from build123d import *

# Parameters (mm, degrees)
F1_DEPTH  = 55
F3_DEPTH  = 30
F4_R      = 3
F5_DEPTH  = 25
F6_R      = 12.5
F7_DEPTH  = 25
F8_R      = 15.1
F9_DEPTH  = 38
F10_R     = 15.1
F11_DEPTH = 8
F12_R     = 6.5
F13_DEPTH = 17
F14_R     = 10


with BuildPart() as f1:
    # F0 (on Front) → F1 (new body)
    with BuildSketch(Plane.XZ):
        with BuildLine():
            Line((-23.699999, 23.799999), (-23.699999, 23.558845))
            Line((-23.699999, 23.558845), (-24.369059, 22.399999))
            Line((-24.369059, 22.399999), (-23.699999, 21.241153))
            Line((-23.699999, 21.241153), (-23.699999, -21.000001))
            ThreePointArc((-23.699999, -21.000001), (-22.001218, -25.10122), (-17.899999, -26.8))
            Line((-17.899999, -26.8), (15.100001, -26.8))
            ThreePointArc((15.100001, -26.8), (19.20122, -25.10122), (20.9, -21.000001))
            Line((20.9, -21.000001), (20.9, -4.000001))
            ThreePointArc((20.9, -4.000001), (21.251472, -3.151472), (22.100001, -2.8))
            Line((22.100001, -2.8), (22.9, -2.8))
            Line((22.9, -2.8), (22.9, 2.799999))
            Line((22.9, 2.799999), (22.100001, 2.799999))
            ThreePointArc((22.100001, 2.799999), (21.251472, 3.151471), (20.9, 3.999999))
            Line((20.9, 3.999999), (20.9, 11.499999))
            ThreePointArc((20.9, 11.499999), (21.397919, 12.702081), (22.600001, 13.2))
            Line((22.600001, 13.2), (23.100001, 13.2))
            ThreePointArc((23.100001, 13.2), (23.665686, 13.434314), (23.9, 13.999999))
            Line((23.9, 13.999999), (23.9, 21.241153))
            Line((23.9, 21.241153), (24.56906, 22.399999))
            Line((24.56906, 22.399999), (23.9, 23.558845))
            Line((23.9, 23.558845), (23.9, 23.799999))
            Line((23.9, 23.799999), (-23.699999, 23.799999))
        make_face()
    extrude(amount=F1_DEPTH)

    # F2 (on face) → F3 (cut)
    with BuildSketch(Plane.XZ.offset(55)):
        with BuildLine():
            Line((15.9, 11.457851), (26.682628, 11.457851))
            Line((26.682628, 11.457851), (26.682628, 26.709846))
            Line((26.682628, 26.709846), (-26.825872, 26.709846))
            Line((-26.825872, 26.709846), (-26.825872, -17.8))
            Line((-26.825872, -17.8), (5.9, -17.8))
            Line((5.9, -17.8), (10.9, -17.8))
            Line((10.9, -17.8), (10.9, -11.8))
            Line((10.9, -11.8), (10.9, 6.457851))
            ThreePointArc((10.9, 6.457851), (12.364466, 9.993385), (15.9, 11.457851))
        make_face()
    extrude(amount=-F3_DEPTH, mode=Mode.SUBTRACT)

    # F4 (on face) → F5 (cut)
    with BuildSketch(Plane.YZ.offset(22.9)):
        with Locations((-48, -1e-06)):
            Circle(F4_R)
        with Locations((-32, -1e-06)):
            Circle(F4_R)
    extrude(amount=-F5_DEPTH, mode=Mode.SUBTRACT)

    # F6 (on face) → F7 (cut, through all)
    with BuildSketch(Plane(origin=(0, 0, 0), x_dir=(-1, 0, 0), z_dir=(0, 1, 0))):
        with Locations((5.799999, -0.9)):
            Circle(F6_R)
    extrude(amount=-F7_DEPTH, mode=Mode.SUBTRACT)

    # F8 (on face) → F9 (cut)
    with BuildSketch(Plane.XZ.offset(55)):
        with Locations((-5.799999, -0.9)):
            Circle(F8_R)
    extrude(amount=-F9_DEPTH, mode=Mode.SUBTRACT)

    # F10 (on face) → F11 (cut)
    with BuildSketch(Plane(origin=(0, 0, 0), x_dir=(-1, 0, 0), z_dir=(0, 1, 0))):
        with Locations((5.799999, -0.9)):
            Circle(F10_R)
    extrude(amount=-F11_DEPTH, mode=Mode.SUBTRACT)

    # F12 (on Right) → F13 (cut)
    with BuildSketch(Plane.YZ):
        with Locations((-32, 0)):
            Circle(F12_R)
        with Locations((-48, 0)):
            Circle(F12_R)
    extrude(amount=F13_DEPTH, mode=Mode.SUBTRACT)

    # F14
    f14_edges = [f1.edges().sort_by_distance(p)[0] for p in [
        (10.9, -40, -17.8),
    ]]
    fillet(f14_edges, radius=F14_R)


solid = f1.part
Source: CAD feature listing. Evaluate the final solid. Frame: model axes, mm. A direction names the side the tool comes from. Round coordinates to 2 decimals unless told otherwise and drop trailing zeros. Write each loop counter-clockwise with the first axis right and the second up, starting at its lowest first coordinate (ties: lowest second). Pieces come first, ordered by that corner, then holes. Notation, with made-up numbers: (88.5, 73) - (120.5, 73) arc R27 ccw to (120.5, 107) - close; hole circle Ø1 at (86, 69.25). An arc over 180 degrees is marked (long way). Use CSV: the item, a comma, the result in double quotes. Start each with the question number.
(1) Cut plane A-A, the plane y = -20. Return loops of the section in (x, z).
(2) First-contact query: pin 1 Ø21 at (y, z) = (-32.5, 1) entering from -X; pin 2 Ø3 at (y, z) = (-8, -1) entering from +X; pin 3 Ø11.5 at (y, z) = (-48, 0) entering from -X. Flat tips, straight axial feed; report the tip coordinate or a pass-through.
(3) Cut plane D-D, the plane z = -10.5. Return loops of the section in (x, y), and give its area (3 significant figures).
(4) Material intervals for probe 1 along Y at (x, z) = (13.75, 0); probe 2 along Z at (x, y) = (-15, -47.5); probe 3 along X at (y, z) = (-13.5, 17.5), sorted ascending. Write a range as [from, to].
(5) Mould query, pull axis Z, two halves, no side actions, for faces 4 (the face through (0, -12, 23.8)), 5 (the face through (10.9, -40, -2)), 6 (the face through (13.907, -54.494, 0.286)). Classes: pulls with the +Z half, pulls with the -Z half, needs draft (parallel to the pull), parting line crosses it, or undercut.
(6) Cut plane B-B, the plane z = 0. Give the number of separate pieces and of enclosed holes in the cut face, and give its area (3 significant figures).
(7) Cut plane C-C, the plane x = -3. Return loops of the section in (y, z).
(8) Set-up query: faces 1 (the face through (8.05, -39.79, -14.79)), 2 (the face through (13.907, -38.494, 0.286)), 3 (the face through (-11.5, -17, 10.4)). Return all of +Z, -Z, +X, -X, +Y, -Y with unobstructed straight access to the full face (end or side cutting, diameter ignored); none if empty.
Geometry says:
1,outline,"(-24.37, 22.4) - (-23.7, 21.24) - (-23.7, -21) arc R5.8 ccw to (-17.9, -26.8) - (15.1, -26.8) arc R5.8 ccw to (20.9, -21) - (20.9, -4) arc R1.2 cw to (22.1, -2.8) - (22.9, -2.8) - (22.9, 2.8) - (22.1, 2.8) arc R1.2 cw to (20.9, 4) - (20.9, 11.5) arc R1.7 cw to (22.6, 13.2) - (23.1, 13.2) arc R0.8 ccw to (23.9, 14) - (23.9, 21.24) - (24.57, 22.4) - (23.9, 23.56) - (23.9, 23.8) - (-23.7, 23.8) - (-23.7, 23.56) - close; hole circle Ø30.2 at (-5.8, -0.9)"
2,pin 1,"x = -23.7"
2,pin 2,"x = 22.9"
2,pin 3,"x = 17"
3,outline,"(-23.7, -25) - (-17.46, -25) - (-17.46, -17) - (-13.81, -17) - (-13.81, -8) - (-17.46, -8) - (-17.46, 0) - (-23.7, 0) - close; (2.21, -17) - (5.86, -17) - (5.86, -25) - (10.53, -25) - (10.53, -55) - (20.9, -55) - (20.9, 0) - (5.86, 0) - (5.86, -8) - (2.21, -8) - close"
3,area,"909 mm²"
4,probe 1,"[-55, -54.5], [-41.5, -38.5], [-25.5, 0]"
4,probe 2,"[-26.8, -17.8]"
4,probe 3,"[-23.7, 23.9]"
5,face 4,"pulls with the +Z half"
5,face 5,"needs draft"
5,face 6,"undercut"
6,separate pieces,"4"
6,enclosed holes,"0"
6,area,"589 mm²"
7,outline,"(-55, -26.8) - (0, -26.8) - (0, -15.74) - (-8, -15.74) - (-8, -13.08) - (-17, -13.08) - (-17, -15.74) - (-25, -15.74) - (-25, -17.8) - (-55, -17.8) - close; (-25, 13.94) - (-17, 13.94) - (-17, 11.28) - (-8, 11.28) - (-8, 13.94) - (0, 13.94) - (0, 23.8) - (-25, 23.8) - close"
8,face 1,"+Z, -X, -Y"
8,face 2,"-X"
8,face 3,"-Y"
